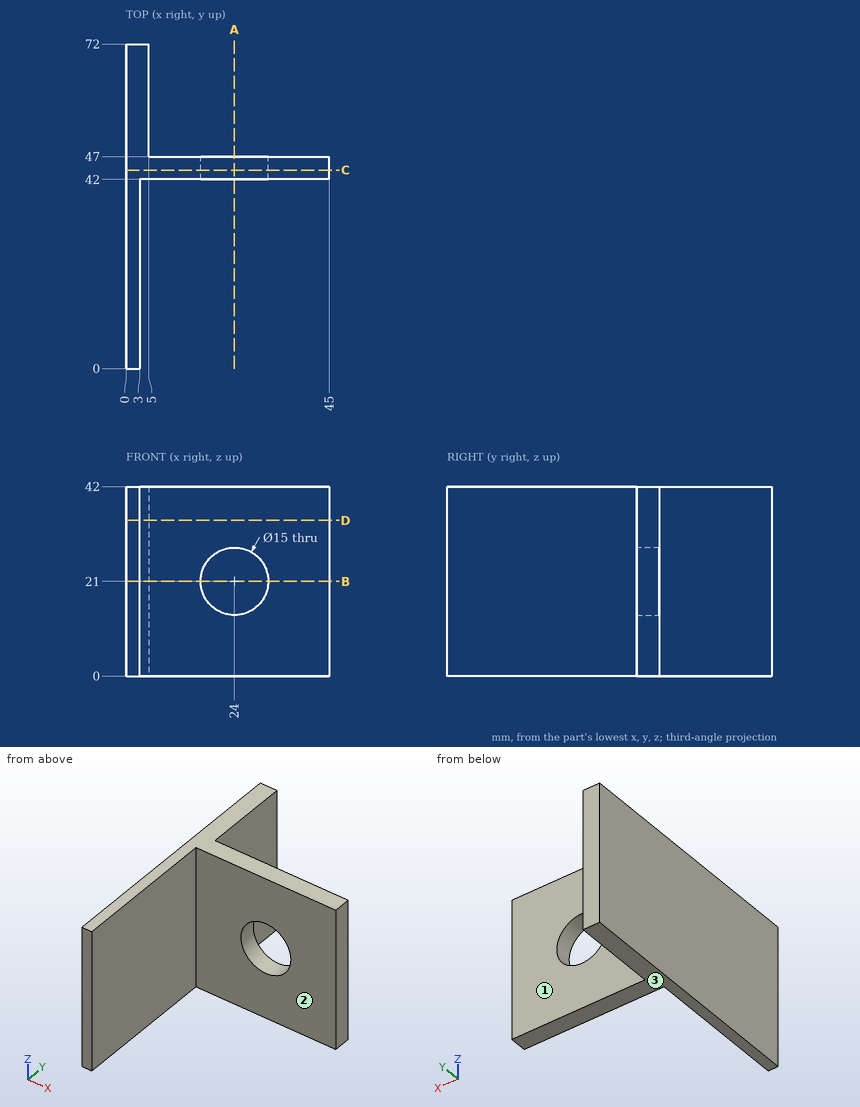
Geometry check sheet. Reference: drawing and pictorial views, mm from the part's lowest x, y, z. A direction names the side the tool comes from. Coordinates: 2 decimals unless noted, no trailing zeros. Loops run counter-clockwise (first coordinate to the right, second up) from the corner with the lowest first, then second, coordinate; pieces in that order, holes last. Notation, with made-up numbers: (56, 61) -> (62, 61) arc R20 cw to (62, 93) -> close; hole circle Ø7 at (-13, -11). An arc over 180 degrees is marked (long way). Put each result on its own line as item: value.
1) Cross-section at D-D on z = 34.5. Record the boundary of the cut face in (x, y).
Result set:
outline: (0, 0) -> (3, 0) -> (3, 42) -> (45, 42) -> (45, 47) -> (5, 47) -> (5, 72) -> (0, 72) -> close
2) Cross-section at A-A on x = 24. Record the boundary of the cut face in (y, z), plus the area to 3 significant figures.
Result set:
outline: (42, 0) -> (47, 0) -> (47, 13.5) -> (42, 13.5) -> close; (42, 28.5) -> (47, 28.5) -> (47, 42) -> (42, 42) -> close
area: 135 mm^2
3) Gauge pin test, flat ends, axial feed: pin 1 Ø8 at (y, z) = (60, 12.5) entering from +X; pin 2 Ø5 at (x, z) = (6.5, 10.5) entering from -Y; pin 3 Ø20 at (x, z) = (35, 29) entering from +Y. Record the tip position at first contact, or that the pin passes through.
Result set:
pin 1: stops at x = 5
pin 2: stops at y = 42
pin 3: stops at y = 47
4) Thickness scan on line 1 (X direction, y = 43, z = 21); line 2 (X direction, y = 19, z = 3.5); line 3 (X direction, y = 61.5, z = 33). Record the ranges inside material, lowest first.
Result set:
line 1: x = 0 to 16.5, 31.5 to 45
line 2: x = 0 to 3
line 3: x = 0 to 5
5) Cross-section at B-B on z = 21. Record the boundary of the cut face in (x, y), plus the area to 3 significant figures.
Result set:
outline: (0, 0) -> (3, 0) -> (3, 42) -> (16.5, 42) -> (16.5, 47) -> (5, 47) -> (5, 72) -> (0, 72) -> close; (31.5, 42) -> (45, 42) -> (45, 47) -> (31.5, 47) -> close
area: 401 mm^2
6) Cross-section at C-C on y = 44. Record the boundary of the cut face in (x, z), plus the area to 3 significant figures.
Result set:
outline: (0, 0) -> (45, 0) -> (45, 42) -> (0, 42) -> close; hole circle Ø15 at (24, 21)
area: 1,710 mm^2
7) Tool access check on the marked faces 1, 2 and 3. Record the directions out of +Z, -Z, +X, -X, +Y, -Y that give a thin tool (end or side, any length) a straight path to the whole face; none if there is none.
Result set:
face 1: +Z, -Z, +X, +Y
face 2: +Z, -Z, +X, -Y
face 3: -Z, +X, -X, +Y, -Y
